Source: CAD feature listing. Evaluate the final solid. Frame: model axes, mm. Give positions to 0.01 mm unless a question says otherwise; leave off trailing zeros. Loops run counter-clockwise (first coordinate to the right, second up) from the corner with the lowest first, then second, coordinate; pieces in that order, holes last. Notation, with made-up numbers: M -12,12 L 47,12 A11 ccw 47,31 Z; hole C 68,76.5 d4. An arc over 180 degrees is marked long. Answer in a Markdown table with one row per item.
```python
from build123d import *

# Parameters (mm, degrees)
F0_W     = 77.6591151953
F0_H     = 11.8106603622
F1_DEPTH = 101.6
F2_DEPTH = 38.989
F3_DEPTH = 1.4478
F4_DEPTH = 50.8
F5_R     = 50.8
F7_D     = 25.4


with BuildPart() as f1:
    # F0 (on Front) → F1 (new body)
    with BuildSketch(Plane.XZ):
        with Locations((38.8295575976, 5.9053301811)):
            Rectangle(F0_W, F0_H)
    extrude(amount=F1_DEPTH)

    # F2 (add): a face of the model
    f2_faces = [f1.faces().sort_by_distance(p)[0] for p in [
        (38.8295575976, -50.8, 11.8106603622),
    ]]
    extrude(f2_faces, amount=F2_DEPTH)

    # F3 (cut): a face of the model
    f3_faces = [f1.faces().sort_by_distance(p)[0] for p in [
        (77.6591151953, -50.8, 25.3998301811),
    ]]
    extrude(f3_faces, amount=-F3_DEPTH, mode=Mode.SUBTRACT)

    # F4 (add): a face of the model
    f4_faces = [f1.faces().sort_by_distance(p)[0] for p in [
        (76.2113151953, -50.8, 25.3998301811),
    ]]
    extrude(f4_faces, amount=F4_DEPTH)

    # F5
    f5_edges = [f1.edges().sort_by_distance(p)[0] for p in [
        (127.011315, 0, 25.39983),
    ]]
    fillet(f5_edges, radius=F5_R)

    # F7 (through all)
    with Locations(Plane(origin=(0, 0, 0), x_dir=(1, 0, 0), z_dir=(0, 0, -1))):
        with Locations((93.4151336551, 30.8703370392)):
            Hole(F7_D / 2)


solid = f1.part
```
Q1. Contact query for a flat-ended pin moving along its axis: pin 1 Ø1 at (x, z) = (113.5, 11.5) entering from +Y. Output: stop coordinate, or through.
Values follow:
| item | result |
|---|---|
| pin 1 | y = -15.77 |
Q2. Section query A-A (y = -29). Output: boundary loops of the cut face in (x, z).
Values follow:
| item | result |
|---|---|
| outline | M 0,0 L 80.85,0 L 80.85,50.8 L 0,50.8 Z; M 105.98,0 L 122.1,0 L 122.1,50.8 L 105.98,50.8 Z |
Q3. Section query B-B (z = 37.5). Output: boundary loops of the cut face in (x, y), plus the area to 3 significant figures.
Values follow:
| item | result |
|---|---|
| outline | M 0,-101.6 L 127.01,-101.6 L 127.01,-50.8 A50.8 ccw 76.21,0 L 0,0 Z; hole C 93.42,-30.87 d25.4 |
| area | 11,800 mm^2 |
Q4. Ray query, probe 1 along X at (y, z) = (-29, 49); probe 2 along X at (y, z) = (-32.5, 21.5); probe 3 along Y at (x, z) = (109, 3). Return the intervals inside material, ascending. Write a range as from..to.
Values follow:
| item | result |
|---|---|
| probe 1 | 0..80.85, 105.98..122.1 |
| probe 2 | 0..80.82, 106.01..123.6 |
| probe 3 | -101.6..-12 |
Q5. Section query C-C (y = -14.5). Output: boundary loops of the cut face in (x, z).
Values follow:
| item | result |
|---|---|
| outline | M 0,0 L 111.75,0 L 111.75,50.8 L 0,50.8 Z |
